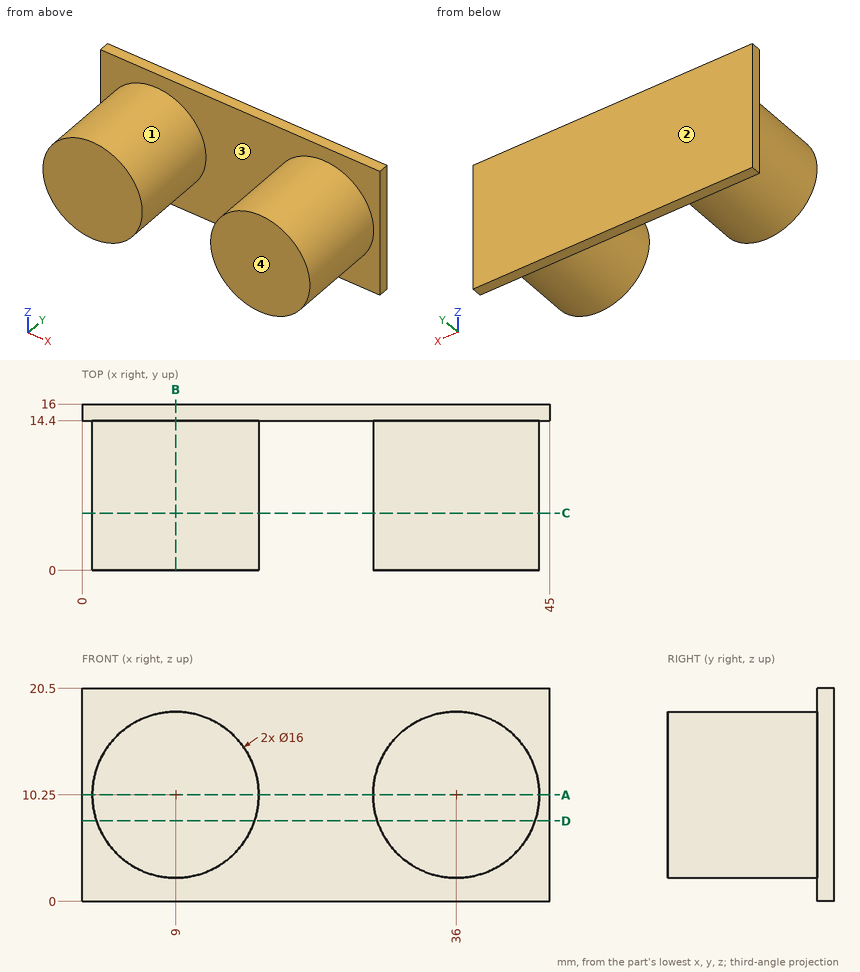
Job drawing, mm, ordinate dimensions from the low corner. One solid piece. A direction names the side the tool comes from. Give positions to 0.01 mm unless a question says otherwise; leave off trailing zeros. Write each loop counter-clockwise with the first axis right and the second up, starting at its lowest first coordinate (ties: lowest second). Pieces come first, ordered by that corner, then holes. Notation, with made-up numbers: (18, -13) - (49, -13) arc R9 cw to (49, -6) - close; hole circle Ø11 at (83, 78). An arc over 180 degrees is marked (long way). Use one line per item in the form item = value. Start each with the question number.
1. 3-axis set-ups, long thin cutter, end or side, ignore diameter. For the marked faces 3 and 4: which of +Z, -Z, +X, -X, +Y, -Y reach the whole face in a straight line?
2. Two-plate mould, pull along X, no slides. Class the marked faces 1 and 2: released by +X, released by -X, zero draft, split by the parting line, or undercut.
3. Band-saw the part on B-B on x = 9. Write the cut outline in (y, z), plus the area to 3 significant figures.
4. Band-saw the part on D-D on z = 7.75. Write the cut outline in (x, y), plus the area to 3 significant figures.
5. Band-saw the part on A-A on z = 10.25. Write the cut outline in (x, y), plus the area to 3 significant figures.
6. Probe line 1 (Z direction, x = 36, y = 5.75); line 2 (X direction, y = 13, z = 4.25); line 3 (Y direction, x = 4.5, z = 2.75). List the from-to ranges inside material, lowest first. Write a range as [from, to].
7. Band-saw the part on C-C on y = 5.5. Write the cut outline in (x, z), plus the area to 3 significant figures.
8. Drop flat-ended pins along their axis: pin 1 Ø4 at (x, y) = (15.5, 2) entering from -Z; pin 2 Ø5 at (x, y) = (31, 2.5) entering from +Z; pin 3 Ø3 at (x, y) = (28, 7) entering from +Z. Give the stop position or say it passes through.
Conclusion:
q1.face_3 = -Y
q1.face_4 = +Z, -Z, +X, -X, -Y
q2.face_1 = undercut
q2.face_2 = zero draft
q3.outline = (0, 2.25) - (14.4, 2.25) - (14.4, 0) - (16, 0) - (16, 20.5) - (14.4, 20.5) - (14.4, 18.25) - (0, 18.25) - close
q3.area = 263 mm²
q4.outline = (0, 14.4) - (1.4, 14.4) - (1.4, 0) - (16.6, 0) - (16.6, 14.4) - (28.4, 14.4) - (28.4, 0) - (43.6, 0) - (43.6, 14.4) - (45, 14.4) - (45, 16) - (0, 16) - close
q4.area = 510 mm²
q5.outline = (0, 14.4) - (1, 14.4) - (1, 0) - (17, 0) - (17, 14.4) - (28, 14.4) - (28, 0) - (44, 0) - (44, 14.4) - (45, 14.4) - (45, 16) - (0, 16) - close
q5.area = 533 mm²
q6.line_1 = [2.25, 18.25]
q6.line_2 = [3.71, 14.29], [30.71, 41.29]
q6.line_3 = [14.4, 16]
q7.outline = circle Ø16 at (9, 10.25); circle Ø16 at (36, 10.25)
q7.area = 402 mm²
q8.pin_1 = 3.64
q8.pin_2 = 17.85
q8.pin_3 = 14.91
